```python
from build123d import *

# Parameters (mm, degrees)
BOSS_EXTRU_1_DEPTH      = 8.75
BOSS_EXTRU_2_DEPTH      = 1
ESQUISSE5_R             = 6
BOSS_EXTRU_3_DEPTH      = 2
ESQUISSE6_R             = 1.5
ENL_V_MAT_EXTRU_1_DEPTH = 0.5
ENL_V_MAT_EXTRU_2_DEPTH = 0.2


with BuildPart() as part:
    # Esquisse2 → Boss.-Extru.1 (new body)
    with BuildSketch(Plane.XY):
        with BuildLine():
            Line((10, 0), (68, 0))
            ThreePointArc((68, 0), (75.071067812, 2.928932188), (78, 10))
            Line((78, 10), (78, 153.4))
            ThreePointArc((78, 153.4), (75.071067812, 160.471067812), (68, 163.4))
            Line((68, 163.4), (10, 163.4))
            ThreePointArc((10, 163.4), (2.928932188, 160.471067812), (0, 153.4))
            Line((0, 153.4), (0, 10))
            ThreePointArc((0, 10), (2.928932188, 2.928932188), (10, 0))
        make_face()
    extrude(amount=BOSS_EXTRU_1_DEPTH)

    # Esquisse4 → Boss.-Extru.2 (add)
    with BuildSketch(Plane.XY.offset(8.75)):
        with BuildLine():
            Line((12.375884012, 159.465412193), (64.375884012, 159.465412193))
            ThreePointArc((64.375884012, 159.465412193), (71.446951823, 156.536480005), (74.375884012, 149.465412193))
            Line((74.375884012, 149.465412193), (74.375884012, 134.465412193))
            ThreePointArc((74.375884012, 134.465412193), (71.446951823, 127.394344381), (64.375884012, 124.465412193))
            Line((64.375884012, 124.465412193), (12.375884012, 124.465412193))
            ThreePointArc((12.375884012, 124.465412193), (5.3048162, 127.394344381), (2.375884012, 134.465412193))
            Line((2.375884012, 134.465412193), (2.375884012, 149.465412193))
            ThreePointArc((2.375884012, 149.465412193), (5.3048162, 156.536480005), (12.375884012, 159.465412193))
        make_face()
    extrude(amount=BOSS_EXTRU_2_DEPTH)

    # Esquisse5 → Boss.-Extru.3 (add)
    with BuildSketch(Plane.XY.offset(9.75)):
        with Locations((12.817579428, 150.680282261)):
            Circle(ESQUISSE5_R)
        with Locations((26.680664603, 142.232464732)):
            Circle(ESQUISSE5_R)
        with Locations((12.817579428, 134.217868615)):
            Circle(ESQUISSE5_R)
    extrude(amount=BOSS_EXTRU_3_DEPTH)

    # Esquisse6 → Enlèv. mat.-Extru.1 (cut)
    with BuildSketch(Plane.XY.offset(9.75)):
        with Locations((66.209801176, 152.964938364)):
            Circle(ESQUISSE6_R)
        with Locations((66.209801176, 131.745411373)):
            Circle(ESQUISSE6_R)
    extrude(amount=-ENL_V_MAT_EXTRU_1_DEPTH, mode=Mode.SUBTRACT)

    # Esquisse9 → Enlèv. mat.-Extru.2 (cut)
    with BuildSketch(Plane.XY.offset(8.75)):
        with BuildLine():
            Line((12.887963043, 116.636129809), (64.887963043, 116.636129809))
            ThreePointArc((64.887963043, 116.636129809), (71.959030855, 113.707197621), (74.887963043, 106.636129809))
            Line((74.887963043, 106.636129809), (74.887963043, 16.636129809))
            ThreePointArc((74.887963043, 16.636129809), (71.959030855, 9.565061997), (64.887963043, 6.636129809))
            Line((64.887963043, 6.636129809), (12.887963043, 6.636129809))
            ThreePointArc((12.887963043, 6.636129809), (5.816895231, 9.565061997), (2.887963043, 16.636129809))
            Line((2.887963043, 16.636129809), (2.887963043, 106.636129809))
            ThreePointArc((2.887963043, 106.636129809), (5.816895231, 113.707197621), (12.887963043, 116.636129809))
        make_face()
    extrude(amount=-ENL_V_MAT_EXTRU_2_DEPTH, mode=Mode.SUBTRACT)


solid = part.part
```
Can you work these out from the model? Positions are in its coordinate system, mm. A direction names the side the tool comes from. Coordinates: 2 decimals unless noted, no trailing zeros. Loops run counter-clockwise (first coordinate to the right, second up) from the corner with the lowest first, then second, coordinate; pieces in that order, holes last. Notation, with made-up numbers: (-24.75, 56.5) -> (-10.75, 56.5) arc R6 cw to (-10.75, 65.5) -> close; hole circle Ø9 at (-23, -35.5). An arc over 180 degrees is marked (long way). Put each result on its own line as item: value. Start each with the question number.
Q1. I want a section at B-B (x = 52). Write out the boundary of the cut face in (y, z).
Q2. For faces 1 (the face through (75.15, 160.39, 4.31)), 2 (the face through (66.01, 154.45, 9.5)), 3 (the face through (71.37, 156.61, 9.24)), which set-ups out of +Z, -Z, +X, -X, +Y, -Y let a thin tool reach every point of the face, with its end or its side?
Q3. I'm going to push flat-ended pins straight in: P1, Ø0.9, axis at x = 66.5, y = 131, coming from the +Z side; P2, Ø1.5, axis at x = 12, y = 50.5, coming from the +Z side; P3, Ø1, axis at x = 44, z = 9.5, coming from the -Y side. Where does each tip first touch, or does it pass through?
Q4. Thinking about a two-plate mould opening in X: for faces 4 (the face through (78, 81, 4)), 5 (the face through (66, 153, 9.25)), 6 (the face through (27, 142, 11.75)), which applies, pulls with the +X half, pulls with the -X half, needs draft (parallel to the pull), parting line crosses it, or undercut?
Q5. I want a section at A-A (y = 38.5). Write out the boundary of the cut face in (x, z), plus the area to 3 significant figures.
Q6. If I drill on line 1 (Z direction, x = 39.5, y = 62.5); line 2 (Y direction, x = 31.5, z = 9.25); line 3 (Z direction, x = 56, y = 151.5), over which ranges is the centre line in solid material (lowest first)? Write a range as [from, to].
Q7. I want a section at C-C (x = 70.5). Write out the boundary of the cut face in (y, z).
Taken from the geometry:
1. outline: (0, 0) -> (163.4, 0) -> (163.4, 8.75) -> (159.47, 8.75) -> (159.47, 9.75) -> (124.47, 9.75) -> (124.47, 8.75) -> (116.64, 8.75) -> (116.64, 8.55) -> (6.64, 8.55) -> (6.64, 8.75) -> (0, 8.75) -> close
2. face 1: +Z, -Z, +X, +Y
2. face 2: +Z
2. face 3: +Z, +X, +Y
3. P1: stops at z = 9.25
3. P2: stops at z = 8.55
3. P3: stops at y = 124.47
4. face 4: pulls with the +X half
4. face 5: undercut
4. face 6: needs draft
5. outline: (0, 0) -> (78, 0) -> (78, 8.75) -> (74.89, 8.75) -> (74.89, 8.55) -> (2.89, 8.55) -> (2.89, 8.75) -> (0, 8.75) -> close
5. area: 668 mm2
6. line 1: z = [0, 8.55]
6. line 2: y = [124.47, 159.47]
6. line 3: z = [0, 9.75]
7. outline: (0.32, 0) -> (163.08, 0) -> (163.08, 8.75) -> (157.37, 8.75) -> (157.37, 9.75) -> (126.56, 9.75) -> (126.56, 8.75) -> (114.91, 8.75) -> (114.91, 8.55) -> (8.36, 8.55) -> (8.36, 8.75) -> (0.32, 8.75) -> close
